Check sheet for the modelled part. Datum: model origin and axes. Units: mm. Face numbers are marked on the shaded views. A direction names the side the tool comes from. Round coordinates to 2 decimals unless told otherwise and drop trailing zeros. Loops run counter-clockwise (first coordinate to the right, second up) from the corner with the lowest first, then second, coordinate; pieces in that order, holes last. Notation, with made-up numbers: (27, 83.5) - (53, 83.5) arc R16 cw to (53, 95.5) - close; hole circle Ø9 at (5, 72). An arc over 180 degrees is marked (long way). Put each result on its own line as item: value. Start each with the question number.
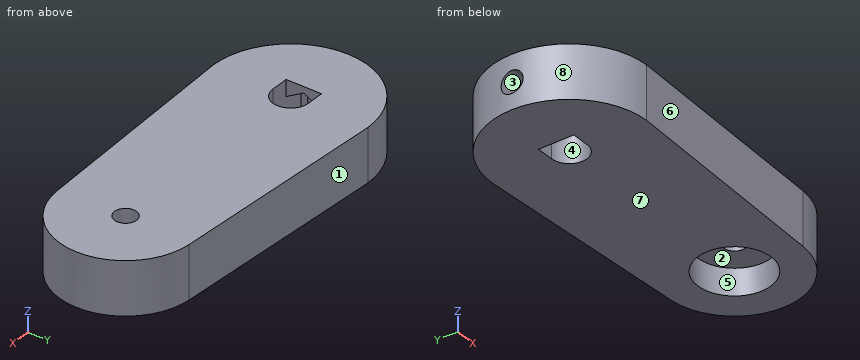
Autodesk Inventor part; units mm, degrees
ref_plane "YZ Plane" through (0, 0, 0) normal (1, 0, 0) x (0, 1, 0)
ref_plane "XZ Plane" through (0, 0, 0) normal (0, 1, 0) x (-1, 0, 0)
ref_plane "XY Plane" through (0, 0, 0) normal (0, 0, 1) x (1, 0, 0)
sketch "Sketch1" plane through (0, 0, 0) normal (0, 0, 1) x (1, 0, 0)
  circle A0 centre (0, 0) radius 4
  arc A1 (0, 17.5) -> (0, -17.5) centre (0, 0) ccw
  arc A2 (50.7435, -14.9816) -> (50.7435, 14.9816) centre (50, 0) ccw
  line L0 (0, 17.5) -> (50.7435, 14.9816)
  line L1 (50.7435, -14.9816) -> (0, -17.5)
  circle A3 centre (50, 0) radius 2.5
  point P0 (1.8995, -17.4057)
  point P1 (1.8995, 17.4057)
  dimension "d0" = 8
  dimension "d1" = 35
  dimension "d2" = 30
  dimension "d3" = 50
  dimension "d4" = 0
  dimension "d5" = 5
extrude "Extrusion1" add sketch "Sketch1" along normal blind 12
sketch "Sketch7" plane through (0, 0, 0) normal (0, 0, -1) x (-1, 0, 0)
  circle A0 centre (-50, 0) radius 2.5
  arc A1 (-50.7435, 14.9816) -> (-50.7435, -14.9816) centre (-50, 0) ccw
  circle A2 centre (-50, 0) radius 8.25
  dimension "d23" = 16.5
extrude "Extrusion7" cut sketch "Sketch7" against normal blind 6
sketch "Sketch8" plane through (0, 0, 12) normal (0, 0, 1) x (1, 0, 0)
  circle A0 centre (0, 0) radius 4
  line L0 (-4, 4) -> (0, 4)
  line L1 (0, 4) -> (0, -4)
  line L2 (0, -4) -> (-4, -4)
  line L3 (-4, -4) -> (-4, 4)
  dimension "d26" = 8
  dimension "d27" = 4
extrude "Extrusion8" cut sketch "Sketch8" against normal through all contours L1 A0 | A0 L3 L0 | L2 L3 A0 picked at (-0.5785, -1.2013)
sketch "Sketch9" plane through (-4, -4, 12) normal (1, 0, 0) x (0, 0, -1)
  circle A0 centre (6, 4) radius 2.5
  point P0 (12, 4)
  dimension "d30" = 5
extrude "Extrusion9" cut sketch "Sketch9" against normal through all
sketch "Sketch10" plane through (-4, -4, 12) normal (1, 0, 0) x (0, 0, -1)
  circle A0 centre (6, 4) radius 2.5
  line L0 (1.3812, 4) -> (3.6906, 8)
  line L1 (3.6906, 8) -> (8.3094, 8)
  line L2 (8.3094, 8) -> (10.6188, 4)
  line L3 (10.6188, 4) -> (8.3094, 0)
  line L4 (8.3094, 0) -> (3.6906, 0)
  line L5 (3.6906, 0) -> (1.3812, 4)
  point P0 (12, 4)
  dimension "d33" = 8
extrude "Extrusion10" cut sketch "Sketch10" against normal blind 4.5
properties part number "20013" material "ABS Plastic"
Q1. Cross-section at D-D on x = -11. Enter the section's corners in (y, z), and give its area (3 significant figures).
Q2. Material ranges on line 1 (X direction, y = 0, z = 9); line 2 (X direction, y = 0, z = 10.65); line 3 (Z direction, x = -13.5, y = 0), recorded low to high. Write a range as from..to.
Q3. Cross-section at C-C on z = 6.75. Enter the section's corners in (x, y).
Q4. Depth check by flat-ended pin: pin 1 Ø4 at (y, z) = (14, 3) entering from -X; pin 2 Ø7 at (x, z) = (-5, 4) entering from +Y; pin 3 Ø6 at (y, z) = (6.5, 2) entering from -X. Enter the tip coordinate at first touch or a pass-through.
Q5. Cross-section at A-A on x = 50. Enter the section's corners in (y, z).
Q6. Set-up check for the marked faces 1, 2, 3 and 4: record each of +Z, -Z, +X, -X, +Y, -Y from which the full face is reachable in a straight line by a thin tool's end or side.
Q7. Cross-section at B-B on y = -7. Enter the section's corners in (x, z), and give its area (3 significant figures).
Q8. Draft check along Y on the marked faces 5, 6, 7 and 8. Enter one of: +Y half, -Y half, draft (parallel to the pull), parting line (faces both ways), or undercut.
Answer list:
1. outline: (-13.61, 0) - (13.61, 0) - (13.61, 12) - (-13.61, 12) - close; hole circle Ø5 at (0, 6)
1. area: 307 mm2
2. line 1: x = -17.5..-8.5, 4..47.5, 52.5..65
2. line 2: x = -17.5..-4, 4..47.5, 52.5..65
2. line 3: z = 0..3.5, 8.5..12
3. outline: (-17.34, -2.38) arc R17.5 ccw to (0, -17.5) - (50.74, -14.98) arc R15 ccw to (50.74, 14.98) - (0, 17.5) arc R17.5 ccw to (-17.34, 2.38) - (-8.5, 2.38) - (-8.5, 4) - (0, 4) arc R4 cw to (0, -4) - (-8.5, -4) - (-8.5, -2.38) - close; hole circle Ø5 at (50, 0)
4. pin 1: stops at x = -12.74
4. pin 2: stops at y = 17.44
4. pin 3: stops at x = -17.15
5. outline: (-15.02, 0) - (-8.25, 0) - (-8.25, 6) - (-2.5, 6) - (-2.5, 12) - (-15.02, 12) - close; (2.5, 6) - (8.25, 6) - (8.25, 0) - (15.02, 0) - (15.02, 12) - (2.5, 12) - close
6. face 1: +Z, -Z, +X, +Y
6. face 2: -Z
6. face 3: -X
6. face 4: +Z, -Z
7. outline: (-16.04, 0) - (45.63, 0) - (45.63, 6) - (54.37, 6) - (54.37, 0) - (63.27, 0) - (63.27, 12) - (-16.04, 12) - close
7. area: 899 mm2
8. face 5: undercut
8. face 6: -Y half
8. face 7: draft
8. face 8: parting line
